Source: three-view drawing plus pictorial views. Frame: mm from the lowest corner of the part. A direction names the side the tool comes from. Give positions to 0.01 mm unless a question says otherwise; leave off trailing zeros. Loops run counter-clockwise (first coordinate to the right, second up) from the corner with the lowest first, then second, coordinate; pieces in that order, holes last. Notation, with made-up numbers: (-5.5, 34.5) -> (37.5, 34.5) arc R26 ccw to (37.5, 67.5) -> close; hole circle Ø5 at (6.5, 67). An arc over 180 degrees is marked (long way). Answer in a Markdown table with one row per item. Add a question column.
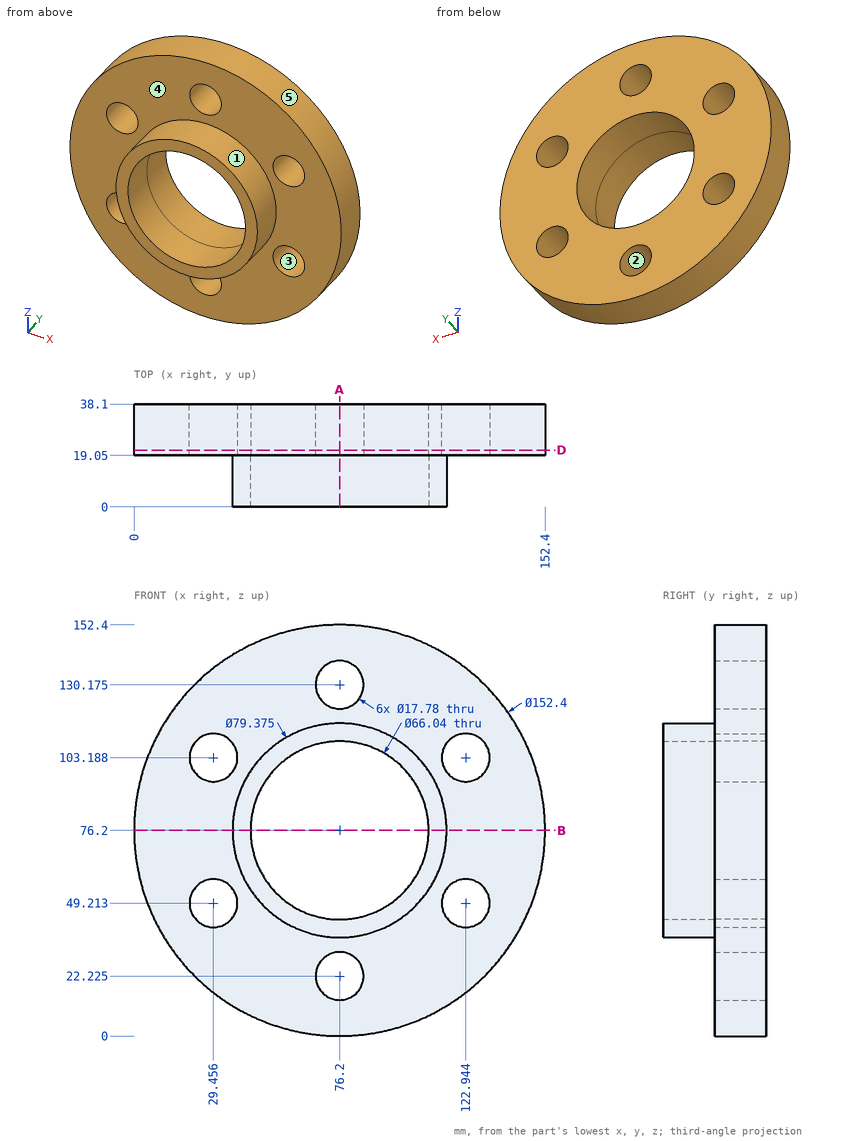
(1) Pin query (flat end, axial travel): pin 1 Ø2 at (x, z) = (128.5, 18.5) entering from +Y; pin 2 Ø12 at (x, y) = (87, 19.5) entering from +Z; pin 3 Ø1.5 at (x, y) = (76, 22) entering from +Z; pin 4 Ø20.5 at (x, z) = (29.46, 49.21) entering from -Y. Return the tip coordinate at first contact, or that it passes through.
(2) Cut plane D-D on y = 21. Return the cut outline in (x, z) (1 decimal).
(3) Cut plane A-A on x = 76.2. State how many separate pieces and enclosed holes the cut face has, then the cut area to 3 significant figures.
(4) Draft query along X for the marked faces 3, 4 and 5. Return one class per face: +X half, -X half, draft (parallel to the pull), parting line (faces both ways), or undercut.
(5) Material intervals for line 1 along Z through (x, y) = (76.2, 25) (1 decimal); line 2 along Y through (x, z) = (135, 33); line 3 along X through (y, z) = (30, 49.5) (1 decimal), sorted ascending. Write a range as from..to.
(6) Reachability of the marked faces 1 and 2 from +Z, -Z, +X, -X, +Y, -Y: full face, straight path, thin tool, end or side. Return the list, or none.
(7) Cut plane B-B on z = 76.2. Return the cut outline in (x, y).
Answer list:
| question | item | result |
|---|---|---|
| 1 | pin 1 | passes through |
| 1 | pin 2 | stops at z = 152.25 |
| 1 | pin 3 | stops at z = 152.4 |
| 1 | pin 4 | stops at y = 19.05 |
| 2 | outline | circle Ø152.4 at (76.2, 76.2); hole circle Ø17.8 at (29.5, 49.2); hole circle Ø17.8 at (29.5, 103.2); hole circle Ø66 at (76.2, 76.2); hole circle Ø17.8 at (76.2, 22.2); hole circle Ø17.8 at (76.2, 130.2); hole circle Ø17.8 at (122.9, 49.2); hole circle Ø17.8 at (122.9, 103.2) |
| 3 | separate pieces | 4 |
| 3 | enclosed holes | 0 |
| 3 | area | 1,220 mm² |
| 4 | face 3 | undercut |
| 4 | face 4 | draft |
| 4 | face 5 | parting line |
| 5 | line 1 | z = 0..13.3, 31.1..43.2, 109.2..121.3, 139.1..152.4 |
| 5 | line 2 | y = 19.05..38.1 |
| 5 | line 3 | x = 4.8..20.6, 38.3..56.8, 95.6..114.1, 131.8..147.6 |
| 6 | face 1 | -Y |
| 6 | face 2 | +Y, -Y |
| 7 | outline | (0, 19.05) -> (36.51, 19.05) -> (36.51, 0) -> (43.18, 0) -> (43.18, 38.1) -> (0, 38.1) -> close; (109.22, 0) -> (115.89, 0) -> (115.89, 19.05) -> (152.4, 19.05) -> (152.4, 38.1) -> (109.22, 38.1) -> close |
